from build123d import *

# Parameters (mm, degrees)
F0_W     = 247.65
F0_H     = 501.65
F1_DEPTH = 19.05
F2_W     = 247.65
F2_H     = 501.65
F2_W_2   = 209.55
F2_H_2   = 463.55
F3_DEPTH = 546.1
F4_W     = 501.65
F4_H     = 19.05
F5_DEPTH = 247.65


with BuildPart() as f1:
    # F0 (on Top) → F1 (new body)
    with BuildSketch(Plane.XY):
        with Locations((-82.35004, 193.778881)):
            Rectangle(F0_W, F0_H)
    extrude(amount=F1_DEPTH)

    # F2 (on face) → F3 (join)
    with BuildSketch(Plane(origin=(0, 0, 0), x_dir=(1, 0, 0), z_dir=(0, 0, -1))):
        with Locations((-82.35004, -193.778881)):
            Rectangle(F2_W, F2_H)
        with Locations((-82.35004, -193.778881)):
            Rectangle(F2_W_2, F2_H_2, mode=Mode.SUBTRACT)
    extrude(amount=F3_DEPTH)

    # F4 (on face) → F5 (join)
    with BuildSketch(Plane(origin=(-206.17504, 0, 0), x_dir=(0, -1, 0), z_dir=(-1, 0, 0))):
        with Locations((-193.778881, -536.575)):
            Rectangle(F4_W, F4_H)
    extrude(amount=-F5_DEPTH)


solid = f1.part
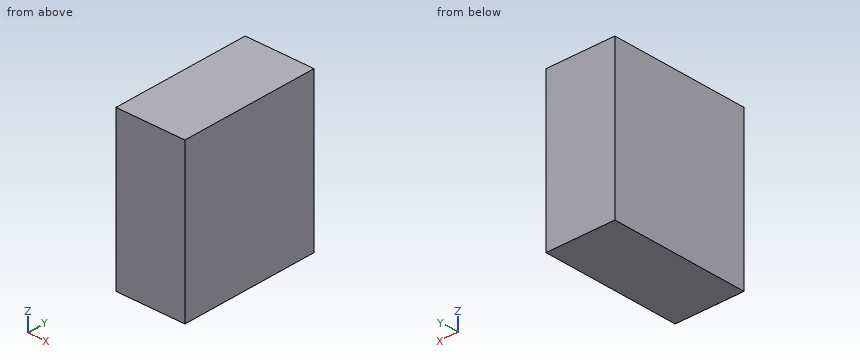
Source: CAD feature listing. Evaluate the final solid. Frame: model axes, mm. Round coordinates to 2 decimals unless told otherwise and drop trailing zeros. Loops run counter-clockwise (first coordinate to the right, second up) from the corner with the lowest first, then second, coordinate; pieces in that order, holes last. Notation, with made-up numbers: M 11,43.5 L 21,43.5 A18 cw 21,55.5 Z; hole C 89,4.5 d7. An arc over 180 degrees is marked long. Return JSON: item names as keys, results as strings. Group by question number.
1. Section query A-A on z = -307.5. Output: boundary loops of the cut face in (x, y), and give its area (3 significant figures).
2. Material intervals for line 1 along Z through (x, y) = (-25.5, 304.5); line 2 along Y through (x, z) = (-68, -172); line 3 along X through (y, z) = (-3, -299), sorted ascending. Write a range as from..to.
3. Section query B-B on y = 351. Output: boundary loops of the cut face in (x, z).
Checks:
{
 "1": {"outline": "M -206.18,-57.05 L 41.47,-57.05 L 41.47,444.6 L -206.18,444.6 Z; hole M -187.13,-38 L 22.42,-38 L 22.42,425.55 L -187.13,425.55 Z", "area": "27,100 mm²"},
 "2": {"line 1": "z = -546.1..-527.05, 0..19.05", "line 2": "y = -57.05..-38, 425.55..444.6", "line 3": "x = -206.18..-187.13, 22.42..41.47"},
 "3": {"outline": "M -206.18,-546.1 L 41.47,-546.1 L 41.47,19.05 L -206.18,19.05 Z; hole M -187.13,-527.05 L 22.42,-527.05 L 22.42,0 L -187.13,0 Z"}
}
